Could you check a few things on this model? Use its own coordinates, in mm. Round coordinates to 2 decimals unless told otherwise and drop trailing zeros. Write each loop counter-clockwise with the first axis right and the second up, starting at its lowest first coordinate (ties: lowest second). Pieces come first, ordered by that corner, then holes. Notation, with made-up numbers: (-8, 48) -> (16, 48) arc R19 ccw to (16, 76) -> close; hole circle Ø4 at (13.5, -27). An arc over 180 degrees is marked (long way). Answer as CSV lines item,"result". Start each with the question number.
Q1. Imagine slicing it at C-C on y = 25.5. Please give me the cut outline in (x, z).
Q2. Imagine slicing it at B-B on y = -176.5. Please give me the cut outline in (x, z).
Q3. Will these pins go through, and if not, where does the flat tip stop? pin 1 Ø1.5 at (y, z) = (-245.5, -172.5) entering from +X; pin 2 Ø20 at (x, y) = (566, -253) entering from +Z; pin 3 Ø1 at (x, y) = (558.5, -64.5) entering from -Z.
Q4. Imagine slicing it at D-D on x = -363.5. Please give me the cut outline in (y, z).
Q5. Imagine slicing it at A-A on z = -8. Please give me the cut outline in (x, y).
Q6. If I drill on line 1 (Z direction, x = 369, y = 54); line 2 (Z direction, x = -550, y = -41); line 3 (X direction, y = 60, z = -17), over which ranges is the centre line in solid material (lowest first)? Write a range as [from, to].
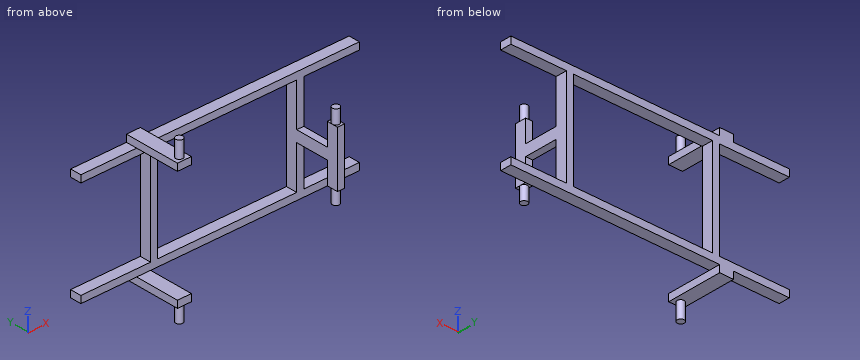
from build123d import *

# Parameters (mm, degrees)
CROQUIS1_W              = 50.8
CROQUIS1_H              = 50.8
CROQUIS1_W_2            = 399.2
CROQUIS1_H_2            = 149.2
CROQUIS1_H_3            = 160
CROQUIS1_H_4            = 80
CROQUIS1_H_5            = 698.4
CROQUIS1_W_3            = 100
SALIENTE_EXTRUIR1_DEPTH = 80
CROQUIS1_4_W            = 100
CROQUIS1_4_H            = 50.8
CROQUIS1_4_W_2          = 50.8
CROQUIS1_4_H_2          = 80
SALIENTE_EXTRUIR2_DEPTH = 320
SALIENTE_EXTRUIR3_START = -320
CROQUIS1_5_W            = 50.8
CROQUIS1_5_H            = 160
CROQUIS1_5_H_2          = 80
SALIENTE_EXTRUIR3_DEPTH = 80
SALIENTE_EXTRUIR4_START = 450.8
CROQUIS2_R              = 25.4
SALIENTE_EXTRUIR4_DEPTH = 120
SALIENTE_EXTRUIR5_START = -570.8
CROQUIS2_7_R            = 25.4
SALIENTE_EXTRUIR5_DEPTH = 120
CROQUIS2_8_R            = 25.4
SALIENTE_EXTRUIR6_DEPTH = 300


with BuildPart() as part:
    # Croquis1 → Saliente-Extruir1 (new body)
    with BuildSketch(Plane(origin=(0, 0, 0), x_dir=(1, 0, 0), z_dir=(0, 1, 0))):
        Polygon((-1000, 400), (-1000, 349.2), (-499.2, 349.2), (-499.2, 400), (-599.2, 400), align=None)
        with Locations((-473.8, 374.6)):
            Rectangle(CROQUIS1_W, CROQUIS1_H)
        Polygon((-448.4, 400), (-448.4, 349.2), (0, 349.2), (550, 349.2), (550, 400), align=None)
        with Locations((800.4, 374.6)):
            Rectangle(CROQUIS1_W_2, CROQUIS1_H)
        with Locations((575.4, 374.6)):
            Rectangle(CROQUIS1_W, CROQUIS1_H)
        with Locations((575.4, 274.6)):
            Rectangle(CROQUIS1_W, CROQUIS1_H_2)
        with Locations((575.4, 120)):
            Rectangle(CROQUIS1_W, CROQUIS1_H_3)
        with Locations((575.4, 0)):
            Rectangle(CROQUIS1_W, CROQUIS1_H_4)
        with Locations((575.4, -120)):
            Rectangle(CROQUIS1_W, CROQUIS1_H_3)
        with Locations((575.4, -274.6)):
            Rectangle(CROQUIS1_W, CROQUIS1_H_2)
        with Locations((575.4, -374.6)):
            Rectangle(CROQUIS1_W, CROQUIS1_H)
        with Locations((800.4, -374.6)):
            Rectangle(CROQUIS1_W_2, CROQUIS1_H)
        Polygon((0, -349.2), (-448.4, -349.2), (-448.4, -400), (550, -400), (550, -349.2), align=None)
        with Locations((-473.8, -374.6)):
            Rectangle(CROQUIS1_W, CROQUIS1_H)
        Polygon((-499.2, -400), (-499.2, -349.2), (-1000, -349.2), (-1000, -400), (-599.2, -400), align=None)
        with Locations((-473.8, 0)):
            Rectangle(CROQUIS1_W, CROQUIS1_H_5)
        with Locations((-549.2, 425.4)):
            Rectangle(CROQUIS1_W_3, CROQUIS1_H)
        with Locations((-549.2, -425.4)):
            Rectangle(CROQUIS1_W_3, CROQUIS1_H)
    extrude(amount=SALIENTE_EXTRUIR1_DEPTH)

    # Croquis1<4> → Saliente-Extruir2 (add)
    with BuildSketch(Plane(origin=(0, 0, 0), x_dir=(1, 0, 0), z_dir=(0, 1, 0))):
        with Locations((-549.2, -425.4)):
            Rectangle(CROQUIS1_4_W, CROQUIS1_4_H)
        with Locations((-549.2, 425.4)):
            Rectangle(CROQUIS1_4_W, CROQUIS1_4_H)
        with Locations((575.4, 0)):
            Rectangle(CROQUIS1_4_W_2, CROQUIS1_4_H_2)
    extrude(amount=-SALIENTE_EXTRUIR2_DEPTH)

    # Croquis1<5> → Saliente-Extruir3 (add)
    with BuildSketch(Plane(origin=(0, 0, 0), x_dir=(1, 0, 0), z_dir=(0, 1, 0)).offset(SALIENTE_EXTRUIR3_START)):
        with Locations((575.4, -120)):
            Rectangle(CROQUIS1_5_W, CROQUIS1_5_H)
        with Locations((575.4, 0)):
            Rectangle(CROQUIS1_5_W, CROQUIS1_5_H_2)
        with Locations((575.4, 120)):
            Rectangle(CROQUIS1_5_W, CROQUIS1_5_H)
    extrude(amount=SALIENTE_EXTRUIR3_DEPTH)

    # Croquis2 → Saliente-Extruir4 (add)
    with BuildSketch(Plane.XY.offset(SALIENTE_EXTRUIR4_START)):
        with Locations((-549.2, -280)):
            Circle(CROQUIS2_R)
    extrude(amount=SALIENTE_EXTRUIR4_DEPTH)

    # Croquis2<7> → Saliente-Extruir5 (add)
    with BuildSketch(Plane.XY.offset(SALIENTE_EXTRUIR5_START)):
        with Locations((-549.2, -280)):
            Circle(CROQUIS2_7_R)
    extrude(amount=SALIENTE_EXTRUIR5_DEPTH)

    # Croquis2<8> → Saliente-Extruir6 (add, symmetric)
    with BuildSketch(Plane.XY):
        with Locations((575.4, -280)):
            Circle(CROQUIS2_8_R)
    extrude(amount=SALIENTE_EXTRUIR6_DEPTH, both=True)


solid = part.part
Checks:
1,outline,"(-1000, -400) -> (-599.2, -400) -> (-599.2, -450.8) -> (-499.2, -450.8) -> (-499.2, -400) -> (1000, -400) -> (1000, -349.2) -> (600.8, -349.2) -> (600.8, 349.2) -> (1000, 349.2) -> (1000, 400) -> (-499.2, 400) -> (-499.2, 450.8) -> (-599.2, 450.8) -> (-599.2, 400) -> (-1000, 400) -> (-1000, 349.2) -> (-499.2, 349.2) -> (-499.2, -349.2) -> (-1000, -349.2) -> close; hole (-448.4, -349.2) -> (550, -349.2) -> (550, 349.2) -> (-448.4, 349.2) -> close"
2,outline,"(-599.2, -450.8) -> (-499.2, -450.8) -> (-499.2, -400) -> (-599.2, -400) -> close; (-599.2, 400) -> (-499.2, 400) -> (-499.2, 450.8) -> (-599.2, 450.8) -> close; (550, -40) -> (600.8, -40) -> (600.8, 40) -> (550, 40) -> close"
3,pin 1,"x = 600.8"
3,pin 2,"z = 300"
3,pin 3,"z = -40"
4,outline,"(0, -400) -> (80, -400) -> (80, -349.2) -> (0, -349.2) -> close; (0, 349.2) -> (80, 349.2) -> (80, 400) -> (0, 400) -> close"
5,outline,"(-499.2, 0) -> (-448.4, 0) -> (-448.4, 80) -> (-499.2, 80) -> close; (550, -320) -> (600.8, -320) -> (600.8, 80) -> (550, 80) -> close"
6,line 1,"[-400, -349.2], [349.2, 400]"
6,line 2,"[-450.8, -400], [400, 450.8]"
6,line 3,"[-499.2, -448.4], [550, 600.8]"
